Part model, mm, in its own coordinate system. Face numbers are marked on the shaded views. A direction names the side the tool comes from. Give positions to 0.01 mm unless a question says otherwise; leave off trailing zeros. Order: outer loops, then holes, each group sorted by start corner. A loop starts at its lowest first (then second) coordinate and runs counter-clockwise, first axis right, second up. Notation, with made-up numbers: M 0.25,66.25 L 20.25,66.25 A3 ccw 20.25,70.25 Z; hole C -40,-19 d10. An arc over 180 degrees is marked long. One line per question, with ' | ' between items.
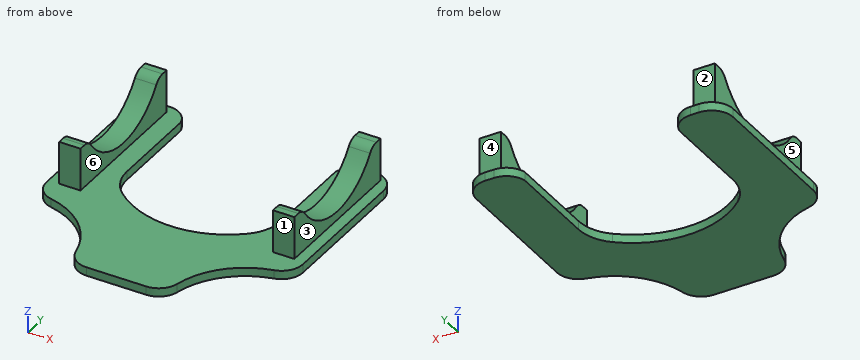
```python
from build123d import *

# Parameters (mm, degrees)
F0_W      = 60
F0_H      = 60
F1_DEPTH  = 2
F2_W      = 5
F2_H      = 34
F3_DEPTH  = 10
F4_R      = 15.85
F5_DEPTH  = 30
F6_R      = 18.5
F7_DEPTH  = 3.5
F8_R      = 5
F10_DEPTH = 4
F11_R     = 10
F12_R     = 3


# Not quite as in the source:
# - a feature names something its author has since deleted; it is built from what else it names


with BuildPart() as f1:
    # F0 (on Top) → F1 (new body)
    with BuildSketch(Plane.XY):
        Rectangle(F0_W, F0_H)
    extrude(amount=-F1_DEPTH)

    # F2 (on face) → F3 (join)
    with BuildSketch(Plane.XY):
        with Locations((-25, 11)):
            Rectangle(F2_W, F2_H)
        with Locations((25, 11)):
            Rectangle(F2_W, F2_H)
    extrude(amount=F3_DEPTH)

    # F4 (on Right) → F5 (cut, symmetric)
    with BuildSketch(Plane.YZ):
        with Locations((10.9725513698, 17.85)):
            Circle(F4_R)
    extrude(amount=F5_DEPTH, both=True, mode=Mode.SUBTRACT)

    # F6 (on Top) → F7 (cut)
    with BuildSketch(Plane.XY):
        with Locations((-29.8706907779, -29.7701153904)):
            Circle(F6_R)
        with Locations((0, 29.9712661654)):
            Circle(F6_R)
        with Locations((30.0718415529, -29.7701153904)):
            Circle(F6_R)
    extrude(amount=-F7_DEPTH, mode=Mode.SUBTRACT)

    # F8
    f8_edges = [f1.edges().sort_by_distance(p)[0] for p in [
        (-30, -11.270567, -1),
        (-11.372119, -30, -1),
        (11.57327, -30, -1),
        (30, -11.270255, -1),
        (30, 30, -1),
        (18.499978, 30, -1),
        (-18.499978, 30, -1),
        (-30, 30, -1),
    ]]
    fillet(f8_edges, radius=F8_R)

    # F9 (on face) → F10 (cut)
    with BuildSketch(Plane.XY):
        with BuildLine():
            Line((18.0813198277, 1.0577162054), (18.0813198277, 26.0577162054))
            ThreePointArc((18.0813198277, 26.0577162054), (0, 11.4712661654), (-18.0813198277, 26.0577162054))
            Line((-18.0813198277, 26.0577162054), (-18.0813198277, 1.0577162054))
            ThreePointArc((-18.0813198277, 1.0577162054), (0, -8.1568370453), (18.0813198277, 1.0577162054))
        make_face()
    extrude(amount=-F10_DEPTH, mode=Mode.SUBTRACT)

    # F11
    f11_edges = [f1.edges().sort_by_distance(p)[0] for p in [
        (-18.08132, 1.057716, -1),
        (18.08132, 1.057716, -1),
    ]]
    fillet(f11_edges, radius=F11_R)

    # F12
    f12_edges = [f1.edges().sort_by_distance(p)[0] for p in [
        (-25, 24.742083, 10),
        (-25, -2.79698, 10),
        (25, 24.742083, 10),
        (25, -2.79698, 10),
    ]]
    fillet(f12_edges, radius=F12_R)


solid = f1.part
```
1. Slice it at D-D on x = 8.5. Give the cut face in (y, z), then the cut area to 3 significant figures.
Worked out:
outline: M -29.79,-2 L -6.48,-2 L -6.48,0 L -29.79,0 Z | area: 46.6 mm2
2. Tool access for the marked faces 1, 2 and 3: list every direction of +Z, -Z, +X, -X, +Y, -Y with a clear straight run to the whole face (end or side of a thin tool).
Worked out:
face 1: +Z, +X, -X, -Y | face 2: +Z, +X, -X, +Y | face 3: +Z, +X, +Y, -Y
3. Slice it at C-C on y = 7.5. Give the cut face in (x, z).
Worked out:
outline: M -30,-2 L -18.08,-2 L -18.08,0 L -22.5,0 L -22.5,2.39 L -27.5,2.39 L -27.5,0 L -30,0 Z; M 18.08,-2 L 30,-2 L 30,0 L 27.5,0 L 27.5,2.39 L 22.5,2.39 L 22.5,0 L 18.08,0 Z
4. Drop flat-ended pins along their axis: pin 1 (3 mm diameter, centred on y = -5, z = 4.5, fed in from -X); pin 2 (5 mm diameter, centred on y = 3, z = 6.5, fed in from +X); pin 3 (2.5 mm diameter, centred on x = 25, z = 6.5, fed in from -Y). Give the stop position or say it passes through.
Worked out:
pin 1: stops at x = -27.5 | pin 2: stops at x = 27.5 | pin 3: stops at y = -6
5. Slice it at B-B on y = 1. Give the cut face in (x, z).
Worked out:
outline: M -30,-2 L -17.31,-2 L -17.31,0 L -22.5,0 L -22.5,5.53 L -27.5,5.53 L -27.5,0 L -30,0 Z; M 17.31,-2 L 30,-2 L 30,0 L 27.5,0 L 27.5,5.53 L 22.5,5.53 L 22.5,0 L 17.31,0 Z
6. Slice it at A-A on z = 6.75. Give the cut face in (x, y).
Worked out:
outline: M -27.5,-6 L -22.5,-6 L -22.5,-0.34 L -27.5,-0.34 Z; M -27.5,22.29 L -22.5,22.29 L -22.5,28 L -27.5,28 Z; M 22.5,-6 L 27.5,-6 L 27.5,-0.34 L 22.5,-0.34 Z; M 22.5,22.29 L 27.5,22.29 L 27.5,28 L 22.5,28 Z
7. Probe L1, parallel to X at y = 25, z = 2.5; L2, parallel to Z at x = -19.5, y = 20.5; L3, parallel to Y at x = -20, z = -1.5. List the from-to ranges inside material, lowest first. Write a range as from..to.
Worked out:
L1: x = -27.5..-22.5, 22.5..27.5 | L2: z = -2..0 | L3: y = -14.12..29.02
8. Mould opens along X. For the marked faces 4, 5 and 6 say: released by +X, released by -X, zero draft, split by the parting line, or undercut.
Worked out:
face 4: zero draft | face 5: released by -X | face 6: undercut
